from build123d import *

# Parameters (mm, degrees)
F0_R     = 10
F1_DEPTH = 5
F2_DEPTH = 5
F3_DEPTH = 2.5


with BuildPart() as f1:
    # F0 (on Right) → F1 (new body, symmetric)
    with BuildSketch(Plane.YZ):
        Circle(F0_R)
        with BuildLine():
            ThreePointArc((14.492753, -6.779388), (15.618644, -3.472459), (16, 0))
            ThreePointArc((16, 0), (15.618644, 3.472459), (14.492753, 6.779388))
            ThreePointArc((14.492753, 6.779388), (-16, 0), (14.492753, -6.779388))
        make_face()
        Circle(F0_R, mode=Mode.SUBTRACT)
    extrude(amount=F1_DEPTH, both=True)

    # F0 (on Right) → F2 (cut, symmetric)
    with BuildSketch(Plane.YZ):
        Circle(F0_R)
    extrude(amount=F2_DEPTH, both=True, mode=Mode.SUBTRACT)

    # F0 (on Right) → F3 (join, symmetric)
    with BuildSketch(Plane.YZ):
        with BuildLine():
            ThreePointArc((14.492753, 6.779388), (15.618644, 3.472459), (16, 0))
            ThreePointArc((16, 0), (15.618644, -3.472459), (14.492753, -6.779388))
            Line((14.492753, -6.779388), (25.476259, -4.338609))
            ThreePointArc((25.476259, -4.338609), (39.567862, -19.248166), (59.375, -13.905372))
            ThreePointArc((59.375, -13.905372), (52.5, 0), (59.375, 13.905372))
            ThreePointArc((59.375, 13.905372), (39.567862, 19.248166), (25.476259, 4.338609))
            Line((25.476259, 4.338609), (14.492753, 6.779388))
        make_face()
    extrude(amount=F3_DEPTH, both=True)


solid = f1.part
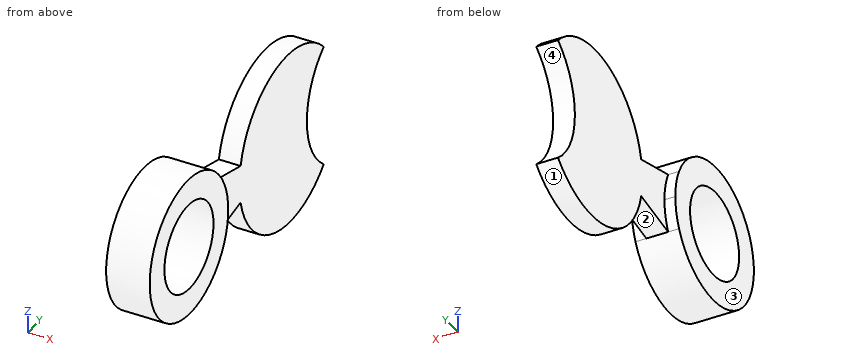
Could you check a few things on this model? Use its own coordinates, in mm. Face numbers are marked on the shaded views. Coordinates: 2 decimals unless noted, no trailing zeros. Write each loop counter-clockwise with the first axis right and the second up, starting at its lowest first coordinate (ties: lowest second). Pieces come first, ordered by that corner, then holes. Notation, with made-up numbers: (82.25, -30.5) - (111.25, -30.5) arc R26 ccw to (111.25, 7.5) - close; hole circle Ø2 at (-26.5, 35.25). An arc over 180 degrees is marked (long way). Write item = value, one per line.
1) Will these pins go through, and if not, where does the flat tip stop? pin 1 Ø4 at (x, z) = (0, 4.5) entering from +Y; pin 2 Ø5 at (x, y) = (-2.5, -2) entering from -Z; pin 3 Ø10 at (y, z) = (42.5, -11.5) entering from -X.
Result set:
pin_1 = 53.75
pin_2 = -16
pin_3 = -2.5
2) Suppose I cut it at C-C on x = 3.5. Please give me the cut outline in (y, z).
Result set:
outline = (14.49, -6.78) arc R16 ccw to (16, 0) arc R16 ccw to (14.49, 6.78) arc R16 ccw (long way) to start; hole circle Ø20 at (0, 0)
3) We'd pull the mould along Y, two halves only. Please class the marked faces 1, 2, 3 and 4: +Y half, -Y half, draft (parallel to the pull), parting line (faces both ways), or undercut.
Result set:
face_1 = undercut
face_2 = undercut
face_3 = draft
face_4 = +Y half
4) Suppose I cut it at B-B on z = 12. Please give me the cut outline in (x, y).
Result set:
outline = (-5, -10.58) - (5, -10.58) - (5, 10.58) - (-5, 10.58) - close; (-2.5, 29) - (2.5, 29) - (2.5, 57.26) - (-2.5, 57.26) - close
5) Suppose I cut it at A-A on y = 0. Please give me the cut outline in (x, z).
Result set:
outline = (-5, -16) - (5, -16) - (5, -10) - (-5, -10) - close; (-5, 10) - (5, 10) - (5, 16) - (-5, 16) - close
6) Please list where these lines run through material, in increasing order: line 1 (Z direction, x = 1.25, y = 0); line 2 (X direction, y = 42, z = -9.5); line 3 (Y direction, x = -1, z = 9). Write a range as [from, to].
Result set:
line_1 = [-16, -10], [10, 16]
line_2 = [-2.5, 2.5]
line_3 = [-13.23, -4.36], [4.36, 13.23], [27.14, 54.99]
